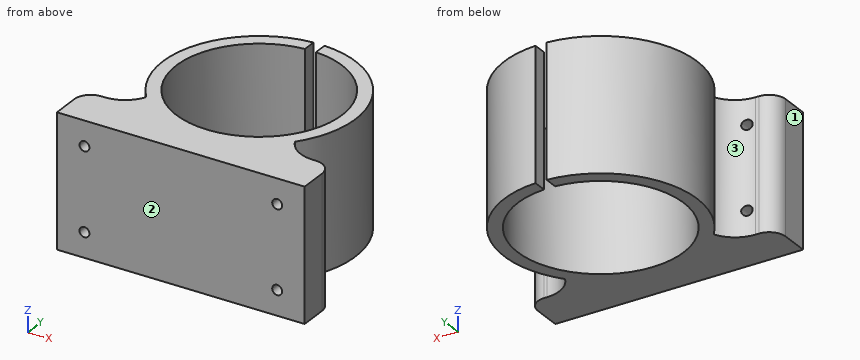
```python
from build123d import *

# Parameters (mm, degrees)
BOSS_EXTRUDE1_DEPTH = 30.48
FILLET1_R           = 7.62
FILLET2_R           = 3.81
CUT_EXTRUDE1_REACH  = 67.853
SKETCH2_R           = 1.143


with BuildPart() as part:
    # Sketch1 → Boss-Extrude1 (new body)
    with BuildSketch(Plane.XY):
        with BuildLine():
            Line((-28.575, 0), (28.575, 0))
            Line((28.575, 0), (28.575, 10.16))
            Line((28.575, 10.16), (17.145, 10.16))
            Line((17.145, 10.16), (17.145, 14.559878518))
            ThreePointArc((17.145, 14.559878518), (20.322966492, 37.697980101), (1.058217697, 50.901792799))
            Line((1.058217697, 50.901792799), (1.058217697, 47.78156187))
            ThreePointArc((1.058217697, 47.78156187), (0.212193658, 9.594292663), (-1.481666667, 47.753356112))
            Line((-1.481666667, 47.753356112), (-1.481666667, 50.877556112))
            ThreePointArc((-1.481666667, 50.877556112), (-20.407880934, 37.503648753), (-17.145, 14.559878518))
            Line((-17.145, 14.559878518), (-17.145, 10.16))
            Line((-17.145, 10.16), (-28.575, 10.16))
            Line((-28.575, 10.16), (-28.575, 0))
        make_face()
    extrude(amount=BOSS_EXTRUDE1_DEPTH)

    # Fillet1
    # the kernel refuses this fillet: 7.62 mm, written as the material it adds along each edge
    with BuildSketch(Plane(origin=(-17.145, 10.16, 0), x_dir=(0, 1, 0), z_dir=(0, 0, 1))) as fillet1_piece_1:
        with BuildLine():
            CenterArc((7.62, 6.906172431), FILLET1_R, 180, 65.001905453)
            Line((0, 6.906172431), (-0.1524, 6.906172431))
            Line((-0.1524, 6.906172431), (-0.1524, 0))
            Line((-0.1524, 0), (0, -0.1524))
            ThreePointArc((0, -0.1524), (2.199939259, -0.1524), (4.335476089, -0.138123449))
            Line((4.335476089, -0.138123449), (4.399878518, 0))
        make_face()
    extrude(amount=30.48)
    with BuildSketch(Plane(origin=(17.145, 10.16, 0), x_dir=(1, 0, 0), z_dir=(0, 0, 1))) as fillet1_piece_2:
        with BuildLine():
            CenterArc((6.906172431, 7.62), FILLET1_R, 204.998094547, 65.001905453)
            Line((0, 4.399878518), (-0.138123449, 4.335476089))
            ThreePointArc((-0.138123449, 4.335476089), (-0.1524, 2.199939259), (-0.1524, 0))
            Line((-0.1524, 0), (0, -0.1524))
            Line((0, -0.1524), (6.906172431, -0.1524))
            Line((6.906172431, -0.1524), (6.906172431, 0))
        make_face()
    extrude(amount=30.48)

    # Fillet2
    fillet2_edges = [part.edges().sort_by_distance(p)[0] for p in [
        (-28.575, 10.16, 15.24),
        (28.575, 10.16, 15.24),
    ]]
    fillet(fillet2_edges, radius=FILLET2_R)

    # Sketch2 → Cut-Extrude1 (cut, up to next)
    with BuildSketch(Plane.XZ, mode=Mode.PRIVATE) as cut_extrude1_sk1:
        with Locations((-22.225, 5.715)):
            Circle(SKETCH2_R)
    cut_extrude1_tool1 = extrude(cut_extrude1_sk1.sketch, amount=-CUT_EXTRUDE1_REACH, mode=Mode.PRIVATE) & part.part
    # Sketch2 → Cut-Extrude1 (cut, up to next)
    with BuildSketch(Plane.XZ, mode=Mode.PRIVATE) as cut_extrude1_sk2:
        with Locations((-22.225, 24.765)):
            Circle(SKETCH2_R)
    cut_extrude1_tool2 = extrude(cut_extrude1_sk2.sketch, amount=-CUT_EXTRUDE1_REACH, mode=Mode.PRIVATE) & part.part
    # Sketch2 → Cut-Extrude1 (cut, up to next)
    with BuildSketch(Plane.XZ, mode=Mode.PRIVATE) as cut_extrude1_sk3:
        with Locations((22.225, 24.765)):
            Circle(SKETCH2_R)
    cut_extrude1_tool3 = extrude(cut_extrude1_sk3.sketch, amount=-CUT_EXTRUDE1_REACH, mode=Mode.PRIVATE) & part.part
    # Sketch2 → Cut-Extrude1 (cut, up to next)
    with BuildSketch(Plane.XZ, mode=Mode.PRIVATE) as cut_extrude1_sk4:
        with Locations((22.225, 5.715)):
            Circle(SKETCH2_R)
    cut_extrude1_tool4 = extrude(cut_extrude1_sk4.sketch, amount=-CUT_EXTRUDE1_REACH, mode=Mode.PRIVATE) & part.part
    add(cut_extrude1_tool1.solids().sort_by_distance((-22.225, 0, 5.715))[0], mode=Mode.SUBTRACT)
    add(cut_extrude1_tool2.solids().sort_by_distance((-22.225, 0, 24.765))[0], mode=Mode.SUBTRACT)
    add(cut_extrude1_tool3.solids().sort_by_distance((22.225, 0, 24.765))[0], mode=Mode.SUBTRACT)
    add(cut_extrude1_tool4.solids().sort_by_distance((22.225, 0, 5.715))[0], mode=Mode.SUBTRACT)


solid = part.part
```
Could you check a few things on this model? Use its own coordinates, in mm. Face numbers are marked on the shaded views. Coordinates: 2 decimals unless noted, no trailing zeros. Order: outer loops, then holes, each group sorted by start corner. A loop starts at its lowest first (then second) coordinate and runs counter-clockwise, first axis right, second up. Notation, with made-up numbers: M -15,-24.75 L 35,-24.75 A30 cw 35,2.25 Z; hole C 16,64 d2. An arc over 180 degrees is marked long. Use one line per item in the form item = value. Start each with the question number.
1. Suppose I cut it at C-C on z = 19.5. Write out the boundary of the cut face in (x, y) (3 decimals), then the cut area to 3 significant figures.
2. Please list where these lines run through material, in increasing order: line 1 (Y direction, x = 6, z = 8); line 2 (Y direction, x = 20, z = 24); line 3 (Y direction, x = 0, z = 17).
3. Suppose I cut it at A-A on y = 41. Write out the boundary of the cut face in (x, z).
4. For pin 1 (3 mm diameter, centred on x = 22.225, z = 5.715, fed in from -Y); pin 2 (3 mm diameter, centred on x = -10.5, z = 22, fed in from +Y); pin 3 (1.5 mm diameter, centred on y = 13, z = 4.5, fed in from +X); pin 4 (0.6 mm diameter, centred on x = 24.5, z = 11.5, fed in from +Y), each with a flat end and sliding along its axis, tell me the tip position at first contact or that it passes through.
5. We'd pull the mould along Y, two halves only. Please class the marked faces 1, 2 and 3: +Y half, -Y half, draft (parallel to the pull), parting line (faces both ways), or undercut.
6. Suppose I cut it at B-B on x = -14. Write out the boundary of the cut face in (y, z).
7. Suppose I cut it at D-D on x = 0. Write out the boundary of the cut face in (y, z).
Geometry says:
q1.outline = M -28.575,0 L 28.575,0 L 28.575,6.35 A3.81 ccw 24.765,10.16 L 24.051,10.16 A7.62 cw 17.145,14.56 A22.225 ccw 1.058,50.902 L 1.058,47.782 A19.109 cw long -1.482,47.753 L -1.482,50.878 A22.225 ccw -17.145,14.56 A7.62 cw -24.051,10.16 L -24.765,10.16 A3.81 ccw -28.575,6.35 Z
q1.area = 946 mm^2
q2.line_1 = 0 to 10.56, 46.84 to 50.1
q2.line_2 = 0 to 11.33, 19.01 to 38.39
q2.line_3 = 0 to 9.59
q3.outline = M -18.51,0 L -14.63,0 L -14.63,30.48 L -18.51,30.48 Z; M 14.63,0 L 18.51,0 L 18.51,30.48 L 14.63,30.48 Z
q4.pin_1 = 0
q4.pin_2 = 49.02
q4.pin_3 = 18.81
q4.pin_4 = 10.16
q5.face_1 = draft
q5.face_2 = -Y half
q5.face_3 = undercut
q6.outline = M 0,0 L 15.7,0 L 15.7,30.48 L 0,30.48 Z; M 41.71,0 L 45.96,0 L 45.96,30.48 L 41.71,30.48 Z
q7.outline = M 0,0 L 9.59,0 L 9.59,30.48 L 0,30.48 Z
